Geometry: final body of the model. Coordinates: model frame, mm. Face numbers are marked on the shaded views. A direction names the side the tool comes from. Give positions to 0.01 mm unless a question says otherwise; leave off trailing zeros. Order: outer loops, then holes, each group sorted by start corner. A loop starts at its lowest first (then second) coordinate and runs counter-clockwise, first axis right, second up. Notation, with made-up numbers: (80.5, 33) - (122.5, 33) arc R20 ccw to (122.5, 49) - close; hole circle Ø10 at (-24, 51.5). An arc over 180 degrees is marked (long way). Use one line per item in the form item = value.
from build123d import *

# Parameters (mm, degrees)
EXTRUDE_1_DEPTH = 100.70048


with BuildPart() as part:
    # 草图2 → 凸台-拉伸1 (new body)
    with BuildSketch(Plane.ZY.offset(123.049709027)):
        Polygon((0, -3.703400415), (0, -8.703400415), (3, -8.703400415), (3, -6.703400415), (8.75, -6.703400415), (8.75, -3.703400415), align=None)
    extrude(amount=-EXTRUDE_1_DEPTH)


solid = part.part
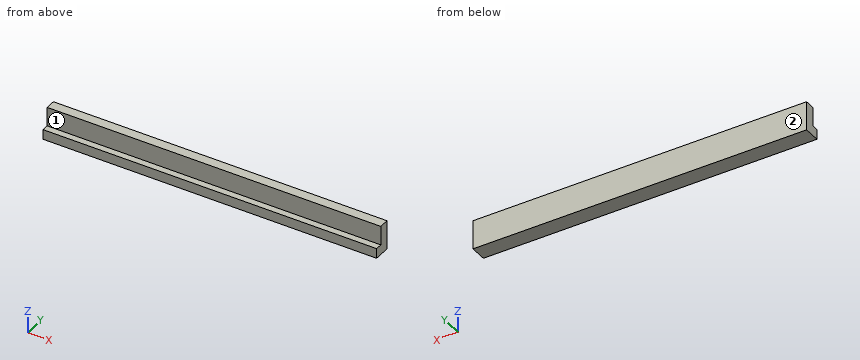
(1) Reachability of the marked faces 1 and 2 from +Z, -Z, +X, -X, +Y, -Y: full face, straight path, thin tool, end or side. Return the list, or none.
Computed values:
face_1 = +Z, +X, -X, -Y
face_2 = +Z, -Z, +X, -X, +Y
(2) Ray query, line 1 along Y through (x, z) = (-87, 8.25); line 2 along Z through (x, y) = (-32.5, -8.3). Return the intervals inside material, ascending.
Computed values:
line_1 = -6.7 to -3.7
line_2 = 0 to 3
(3) Contact query for flat-ended pins moving along their axis: pin 1 Ø0.6 at (x, y) = (-63, -8) entering from +Z; pin 2 Ø3 at (x, z) = (-57.5, 7.5) entering from -Y. Output: stop coordinate, or through.
Computed values:
pin_1 = 3
pin_2 = -6.7
(4) Cut plane C-C on z = 7.75. Output: boundary loops of the cut face in (x, y), plus the area to 3 significant figures.
Computed values:
outline = (-123.05, -6.7) - (-22.35, -6.7) - (-22.35, -3.7) - (-123.05, -3.7) - close
area = 302 mm²
(5) Cut plane A-A on y = -7.75. Output: boundary loops of the cut face in (x, z), plus the area to 3 significant figures.
Computed values:
outline = (-123.05, 0) - (-22.35, 0) - (-22.35, 3) - (-123.05, 3) - close
area = 302 mm²
(6) Cut plane B-B on x = -62.5. Output: boundary loops of the cut face in (y, z).
Computed values:
outline = (-8.7, 0) - (-3.7, 0) - (-3.7, 8.75) - (-6.7, 8.75) - (-6.7, 3) - (-8.7, 3) - close
